Input: part model. Units: mm. Frame: model coordinates. Face numbers are marked on the shaded views. A direction names the side the tool comes from. Give positions to 0.01 mm unless a question says otherwise; leave off trailing zeros. Loops run counter-clockwise (first coordinate to the right, second up) from the corner with the lowest first, then second, coordinate; pieces in that order, holes last. Notation, with made-up numbers: M -31.5,46 L 18.5,46 A20 ccw 18.5,79 Z; hole C -19,50.25 d2. An arc over 180 degrees is marked long. Return JSON: item names as keys, results as strings. Group by question number.
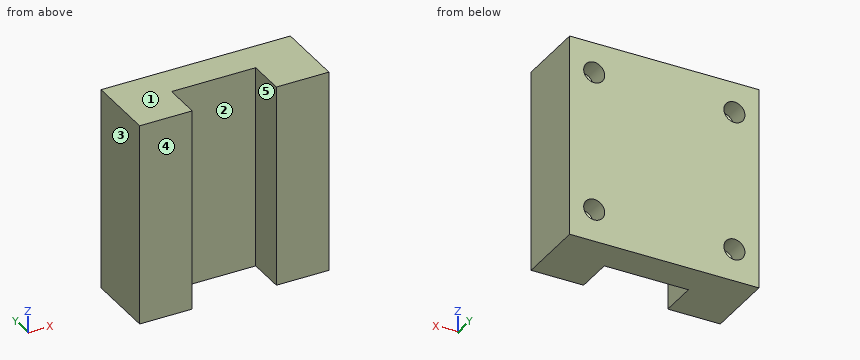
```python
from build123d import *

# Parameters (mm, degrees)
SKETCH1_W                 = 27
SKETCH1_H                 = 28.9
BOSS_EXTRUDE1_DEPTH       = 10
SKETCH2_W                 = 12
SKETCH2_H                 = 5.35
CUT_EXTRUDE1_DEPTH        = 1
CUT_EXTRUDE1_DEPTH_BACK   = 29.9
F_3_0MM_DOWEL_HOLE1_D     = 3
F_3_0MM_DOWEL_HOLE1_DEPTH = 3
F_3_0MM_DOWEL_HOLE1_TIP   = 0.901290929


with BuildPart() as part:
    # Sketch1 → Boss-Extrude1 (new body)
    with BuildSketch(Plane(origin=(0, 0, 0), x_dir=(1, 0, 0), z_dir=(0, 1, 0))):
        with Locations((13.5, 14.45)):
            Rectangle(SKETCH1_W, SKETCH1_H)
    extrude(amount=BOSS_EXTRUDE1_DEPTH)

    # Sketch2 → Cut-Extrude1 (cut, two sides)
    with BuildSketch(Plane.XY) as cut_extrude1_sk:
        with Locations((13.5, 2.675)):
            Rectangle(SKETCH2_W, SKETCH2_H)
    extrude(amount=CUT_EXTRUDE1_DEPTH, mode=Mode.SUBTRACT)
    extrude(cut_extrude1_sk.sketch, amount=-CUT_EXTRUDE1_DEPTH_BACK, mode=Mode.SUBTRACT)

    # Ø3.0mm Dowel Hole1
    with Locations(Plane(origin=(0, 10, 0), x_dir=(1, 0, 0), z_dir=(0, 1, 0))):
        with Locations((3.5, 24.3), (23.5, 24.3), (3.5, 4.3), (23.5, 4.3)):
            Hole(F_3_0MM_DOWEL_HOLE1_D / 2, depth=F_3_0MM_DOWEL_HOLE1_DEPTH)
            with Locations((0, 0, -(F_3_0MM_DOWEL_HOLE1_DEPTH + F_3_0MM_DOWEL_HOLE1_TIP / 2))):  # 118° drill point
                Cone(0, F_3_0MM_DOWEL_HOLE1_D / 2, F_3_0MM_DOWEL_HOLE1_TIP, mode=Mode.SUBTRACT)


solid = part.part
```
Item 1: Material intervals for line 1 (Z direction, x = 23.5, y = 8.55); line 2 (X direction, y = 9, z = -4.3); line 3 (X direction, y = 4, z = -18), sorted ascending. Write a range as from..to.
Item 2: Section A-A, the plane y = 1.5. Return loops of the section in (x, z).
Item 3: Pull-direction query (X, two-part tool) for the marked faces 3, 4 and 5; classes: pulls with the +X half, pulls with the -X half, needs draft (parallel to the pull), parting line crosses it, or undercut.
Item 4: Section B-B, the plane z = -13.5. Return loops of the section in (x, y), then the cut area to 3 significant figures.
Item 5: Reachability of the marked faces 1 and 2 from +Z, -Z, +X, -X, +Y, -Y: full face, straight path, thin tool, end or side. Return the list, or none.
Item 6: Section C-C, the plane x = 14. Return loops of the section in (y, z).
Item 7: First-contact query: pin 1 Ø6 at (x, z) = (15, -11) entering from -Y. Flat tip, straight axial feed; report the tip coordinate or a pass-through.
Answer below:
{
 "1": {"line 1": "-28.9..-25.8, -22.8..-5.8, -2.8..0", "line 2": "0..2, 5..22, 25..27", "line 3": "0..7.5, 19.5..27"},
 "2": {"outline": "M 0,-28.9 L 7.5,-28.9 L 7.5,0 L 0,0 Z; M 19.5,-28.9 L 27,-28.9 L 27,0 L 19.5,0 Z"},
 "3": {"face 3": "pulls with the -X half", "face 4": "needs draft", "face 5": "undercut"},
 "4": {"outline": "M 0,0 L 7.5,0 L 7.5,5.35 L 19.5,5.35 L 19.5,0 L 27,0 L 27,10 L 0,10 Z", "area": "206 mm^2"},
 "5": {"face 1": "+Z, +X, -X, +Y, -Y", "face 2": "+Z, -Z, -Y"},
 "6": {"outline": "M 5.35,-28.9 L 10,-28.9 L 10,0 L 5.35,0 Z"},
 "7": {"pin 1": "y = 5.35"}
}
